Geometry check sheet. Reference: drawing and pictorial views, mm from the part's lowest x, y, z. Round coordinates to 2 decimals unless told otherwise and drop trailing zeros. Loops run counter-clockwise (first coordinate to the right, second up) from the corner with the lowest first, then second, coordinate; pieces in that order, holes last. Notation, with made-up numbers: (18, -34.5) -> (42, -34.5) arc R23 ccw to (42, 4.5) -> close; hole circle Ø4 at (60.25, 54.25). An arc over 180 degrees is marked (long way). Write item = value, one per line.
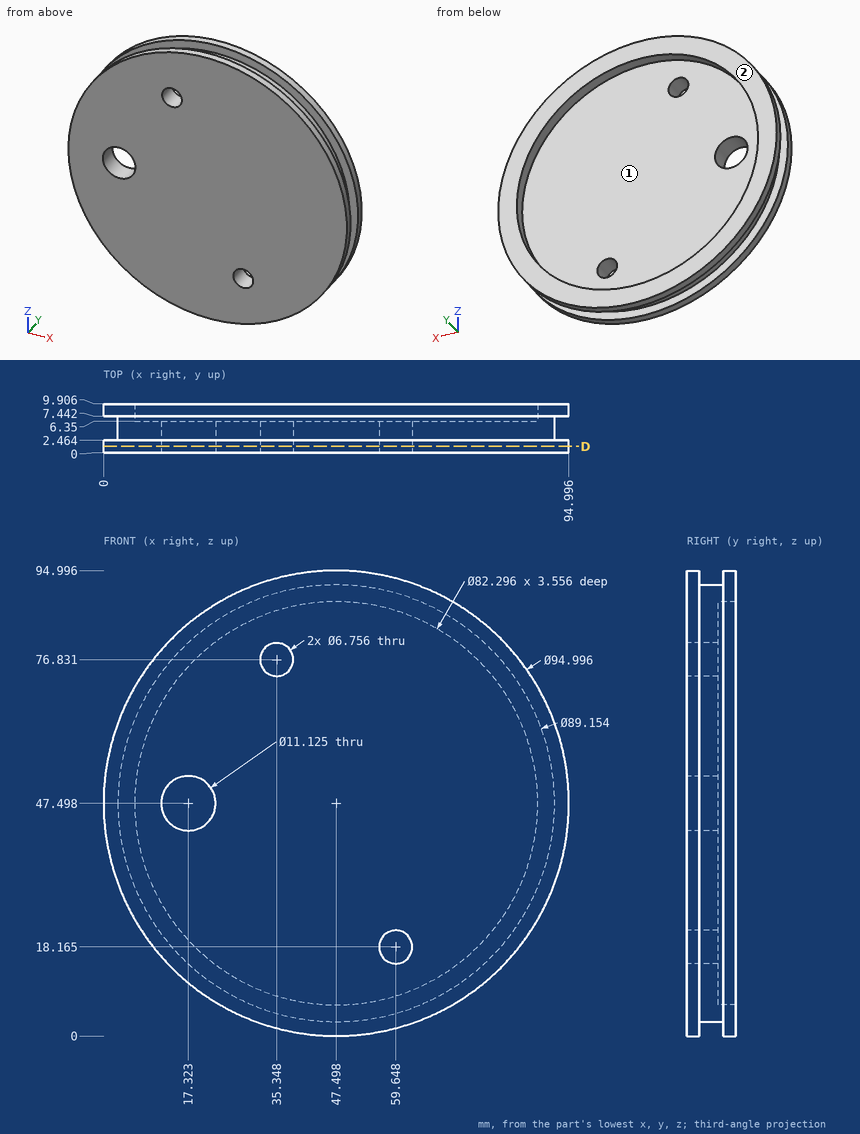
(1) Draft check along Z on the marked faces 1 and 2. Enter one of: released by +Z, released by -Z, zero draft, split by the parting line, or undercut.
Filled sheet:
face_1 = undercut
face_2 = zero draft
(2) Sectioned sample at D-D, the plane y = 1.25. Record the cut outline in (x, z) (1 decimal).
Filled sheet:
outline = circle Ø95 at (47.5, 47.5); hole circle Ø11.1 at (17.3, 47.5); hole circle Ø6.8 at (35.3, 76.8); hole circle Ø6.8 at (59.6, 18.2)
(3) Material ranges on probe 1 along Z at (x, y) = (32, 8) (1 decimal); probe 2 along Y at (x, z) = (35, 14); probe 3 along X at (y, z) = (5.5, 17) (1 decimal), recorded low to high. Write a range as from..to.
Filled sheet:
probe_1 = 2.6..9.4, 85.6..92.4
probe_2 = 0..6.35
probe_3 = 15..56.5, 62.8..80
(4) Go/stop test with flat-tipped pins: pin 1 Ø4 at (y, z) = (2, 57) entering from +X; pin 2 Ø10 at (x, z) = (59.5, 59) entering from -Y; pin 3 Ø2 at (y, z) = (5, 9.5) entering from +X; pin 4 Ø3 at (x, z) = (68.5, 21.5) entering from +Y. Record where each tip stops, or that it passes through.
Filled sheet:
pin_1 = 94.4
pin_2 = 0
pin_3 = 72.36
pin_4 = 6.35
